from build123d import *

# Parameters (mm, degrees)
SKETCH1_R           = 50.8
BOSS_EXTRUDE1_DEPTH = 3.81
CUT_EXTRUDE1_DEPTH  = 72.943005914
SKETCH3_R           = 3.2639
CUT_EXTRUDE2_DEPTH  = 72.943005914
SKETCH4_R           = 4.445
BOSS_EXTRUDE2_DEPTH = 12.7


with BuildPart() as part:
    # Sketch1 → Boss-Extrude1 (new body)
    with BuildSketch(Plane(origin=(0, 0, 0), x_dir=(1, 0, 0), z_dir=(0, 1, 0))):
        with Locations(Location((0, 0, 0), (0, 0, 90))):
            Circle(SKETCH1_R)
    extrude(amount=BOSS_EXTRUDE1_DEPTH)

    # Sketch2 → Cut-Extrude1 (cut, through all)
    with BuildSketch(Plane(origin=(0, 3.81, 0), x_dir=(1, 0, 0), z_dir=(0, 1, 0))):
        with BuildLine():
            ThreePointArc((-13.470384182, 13.470384182), (-7.290119387, 17.599905094), (0, 19.05))
            Line((0, 19.05), (0, 25.4))
            ThreePointArc((0, 25.4), (-9.720159182, 23.466540126), (-17.960512242, 17.960512242))
            Line((-17.960512242, 17.960512242), (-13.470384182, 13.470384182))
        make_face()
        with BuildLine():
            Line((-17.960512242, -17.960512242), (-13.470384182, -13.470384182))
            ThreePointArc((-13.470384182, -13.470384182), (-17.599905094, -7.290119387), (-19.05, 0))
            Line((-19.05, 0), (-25.4, 0))
            ThreePointArc((-25.4, 0), (-23.466540126, -9.720159182), (-17.960512242, -17.960512242))
        make_face()
        with BuildLine():
            Line((17.960512242, -17.960512242), (13.470384182, -13.470384182))
            ThreePointArc((13.470384182, -13.470384182), (7.290119387, -17.599905094), (0, -19.05))
            Line((0, -19.05), (0, -25.4))
            ThreePointArc((0, -25.4), (9.720159182, -23.466540126), (17.960512242, -17.960512242))
        make_face()
        with BuildLine():
            Line((17.960512242, 17.960512242), (13.470384182, 13.470384182))
            ThreePointArc((13.470384182, 13.470384182), (17.599905094, 7.290119387), (19.05, 0))
            Line((19.05, 0), (25.4, 0))
            ThreePointArc((25.4, 0), (23.466540126, 9.720159182), (17.960512242, 17.960512242))
        make_face()
    extrude(amount=-CUT_EXTRUDE1_DEPTH, mode=Mode.SUBTRACT)

    # Sketch3 → Cut-Extrude2 (cut, through all)
    with BuildSketch(Plane(origin=(0, 3.81, 0), x_dir=(1, 0, 0), z_dir=(0, 1, 0))):
        with Locations(Location((13.122214896, 31.67982917, 0), (0, 0, 270))):
            Circle(SKETCH3_R)
        with Locations(Location((24.246691527, 24.246691527, 0), (0, 0, 270))):
            Circle(SKETCH3_R)
        with Locations(Location((31.67982917, 13.122214896, 0), (0, 0, 270))):
            Circle(SKETCH3_R)
        with Locations(Location((31.67982917, -13.122214896, 0), (0, 0, 270))):
            Circle(SKETCH3_R)
        with Locations(Location((24.246691527, -24.246691527, 0), (0, 0, 270))):
            Circle(SKETCH3_R)
        with Locations(Location((13.122214896, -31.67982917, 0), (0, 0, 270))):
            Circle(SKETCH3_R)
        with Locations(Location((0, -34.29, 0), (0, 0, 270))):
            Circle(SKETCH3_R)
        with Locations(Location((-13.122214896, -31.67982917, 0), (0, 0, 270))):
            Circle(SKETCH3_R)
        with Locations(Location((-24.246691527, -24.246691527, 0), (0, 0, 270))):
            Circle(SKETCH3_R)
        with Locations(Location((-31.67982917, -13.122214896, 0), (0, 0, 270))):
            Circle(SKETCH3_R)
        with Locations(Location((-34.29, 0, 0), (0, 0, 270))):
            Circle(SKETCH3_R)
        with Locations(Location((-31.67982917, 13.122214896, 0), (0, 0, 270))):
            Circle(SKETCH3_R)
        with Locations(Location((-24.246691527, 24.246691527, 0), (0, 0, 270))):
            Circle(SKETCH3_R)
        with Locations(Location((-13.122214896, 31.67982917, 0), (0, 0, 270))):
            Circle(SKETCH3_R)
        with Locations(Location((0, 34.29, 0), (0, 0, 270))):
            Circle(SKETCH3_R)
        with Locations(Location((34.29, 0, 0), (0, 0, 270))):
            Circle(SKETCH3_R)
    extrude(amount=-CUT_EXTRUDE2_DEPTH, mode=Mode.SUBTRACT)

    # Sketch4 → Boss-Extrude2 (add)
    with BuildSketch(Plane(origin=(0, 3.81, 0), x_dir=(1, 0, 0), z_dir=(0, 1, 0))):
        Polygon((-6.745760545, 0), (-3.372880273, 5.842), (3.372880273, 5.842), (6.745760545, 0), (3.372880273, -5.842), (-3.372880273, -5.842), align=None)
        with Locations(Location((0, 0, 0), (0, 0, 270))):
            Circle(SKETCH4_R, mode=Mode.SUBTRACT)
    extrude(amount=BOSS_EXTRUDE2_DEPTH)


solid = part.part
Build history of the part. All positions in model axes, mm. A direction names the side the tool comes from. Round coordinates to 2 decimals unless told otherwise and drop trailing zeros. Loops run counter-clockwise (first coordinate to the right, second up) from the corner with the lowest first, then second, coordinate; pieces in that order, holes last. Notation, with made-up numbers: (-18.75, 68.5) -> (13.25, 68.5) arc R12 ccw to (13.25, 76.5) -> close; hole circle Ø3 at (-11, -27.5). An arc over 180 degrees is marked (long way). Use CSV: the item, a comma, the result in double quotes. Start each with the question number.
Q1. Saw through at C-C on x = 41.5. Give the cut face in (y, z), and give its area (3 significant figures).
Q2. Saw through at A-A on y = 11.25. Give the cut face in (x, z) (3 decimals), and give its area (3 significant figures).
Q3. Which spindle directions (+Z, -Z, +X, -X, +Y, -Y) get a long thin tool onto all of the face, cutting with end or side? Do faces 1 (the face through (-4.34, 10.07, -0.96)), 2 (the face through (5.083, 10.071, 2.88)), 3 (the face through (16, 2, 16)), 4 (the face through (-5.083, 10.071, -2.88)). Say none if no direction does.
Q4. Drill centre lines: L1, parallel to X at y = 2.2, z = 34.29; L2, parallel to X at y = 8, z = 0 (3 decimals); L3, parallel to X at y = 2.5, z = -34. Where is each one in solid material? Low to high.
Q5. Saw through at B-B on z = 23.5. Give the cut face in (x, y), and give its area (3 significant figures).
Q6. Flat gauge pins, fed straight in: pin 1 Ø1 at (x, z) = (8.5, -8.5) entering from +Y; pin 2 Ø5.5 at (x, y) = (-0.5, 12.5) entering from -Z; pin 3 Ø1.1 at (y, z) = (2.5, 21) entering from +X; pin 4 Ø3 at (x, z) = (-26.5, -1) entering from -Y. Where does each tip first touch, or does it go through?
Q7. Mould opens along Z. For faces 5 (the face through (-24.103, 1.932, -27.507)), 6 (the face through (-5.036, 10.071, 2.962)), 7 (the face through (-3, 16.51, -3.5)) say: +Z half, -Z half, draft (parallel to the pull), parting line (faces both ways), or undercut.
Solutions:
1,outline,"(0, -29.3) -> (3.81, -29.3) -> (3.81, 29.3) -> (0, 29.3) -> close"
1,area,"223 mm^2"
2,outline,"(-6.746, 0) -> (-3.373, -5.842) -> (3.373, -5.842) -> (6.746, 0) -> (3.373, 5.842) -> (-3.373, 5.842) -> close; hole circle Ø8.89 at (0, 0)"
2,area,"56.2 mm^2"
3,face 1,"+Y"
3,face 2,"+Z, +X, +Y"
3,face 3,"+Y, -Y"
3,face 4,"-Z, -X, +Y"
4,L1,"x = -37.48 to -15.08, -11.16 to -3.26, 3.26 to 11.16, 15.08 to 37.48"
4,L2,"x = -6.746 to -4.445, 4.445 to 6.746"
4,L3,"x = -37.74 to -15.42, -10.83 to -3.25, 3.25 to 10.83, 15.42 to 37.74"
5,outline,"(-45.04, 0) -> (-27.42, 0) -> (-27.42, 3.81) -> (-45.04, 3.81) -> close; (-21.07, 0) -> (0, 0) -> (0, 3.81) -> (-21.07, 3.81) -> close; (9.64, 0) -> (21.07, 0) -> (21.07, 3.81) -> (9.64, 3.81) -> close; (27.42, 0) -> (45.04, 0) -> (45.04, 3.81) -> (27.42, 3.81) -> close"
5,area,"258 mm^2"
6,pin 1,"stops at y = 3.81"
6,pin 2,"stops at z = -5.84"
6,pin 3,"stops at x = 46.5"
6,pin 4,"stops at y = 0"
7,face 5,"undercut"
7,face 6,"+Z half"
7,face 7,"draft"
